from build123d import *

# Parameters (mm, degrees)
BOX035_W          = 6
BOX035_H          = 15
BOX035_DEPTH      = 3
CYLINDER018_R     = 2
CYLINDER018_DEPTH = 50
BOX_W             = 15
BOX_H             = 15
BOX_DEPTH         = 58
BOX038_W          = 80
BOX038_H          = 5
BOX038_DEPTH      = 58
BOX039_W          = 80
BOX039_H          = 90
BOX039_DEPTH      = 4


with BuildPart() as nut_hole:
    # Box035 → Box035 (new body)
    with BuildSketch(Plane(origin=(-8.5, 5, 15), x_dir=(1, 0, 0), z_dir=(0, 0, 1))):
        with Locations((3, 7.5)):
            Rectangle(BOX035_W, BOX035_H)
    extrude(amount=BOX035_DEPTH)


with BuildPart() as cylinder:
    # Cylinder018 → Cylinder018 (new body)
    with BuildSketch(Plane(origin=(-5.5, 12, 0), x_dir=(1, 0, 0), z_dir=(0, 0, 1))):
        Circle(CYLINDER018_R)
    extrude(amount=CYLINDER018_DEPTH)


with BuildPart() as cut:
    # Box → Box (new body)
    with BuildSketch(Plane(origin=(-13, 5, 0), x_dir=(1, 0, 0), z_dir=(0, 0, 1))):
        with Locations((7.5, 7.5)):
            Rectangle(BOX_W, BOX_H)
    extrude(amount=BOX_DEPTH)

    # Cut: cut Cylinder
    add(cylinder.part, mode=Mode.SUBTRACT)


with BuildPart() as cut037:
    # Cut037 base: copy of Cut
    add(cut.part)

    # Cut037: cut Nut hole
    add(nut_hole.part, mode=Mode.SUBTRACT)


with BuildPart() as cut037_1:
    # Cut037 placement: moved
    add(cut037.part.moved(Location((-22, 0, 0))))


with BuildPart() as cut038:
    # Cut038 base: copy of Cut
    add(cut.part)

    # Cut038: cut Nut hole
    add(nut_hole.part, mode=Mode.SUBTRACT)


with BuildPart() as cut038_1:
    # Cut038 placement: moved
    add(cut038.part.moved(Location((43, 0, 0))))


with BuildPart() as extension_supports:
    # Cut039 base: copy of Cut
    add(cut.part)

    # Cut039: cut Nut hole
    add(nut_hole.part, mode=Mode.SUBTRACT)


with BuildPart() as extension_supports_1:
    # Cut039 placement: moved
    add(extension_supports.part.moved(Location((10, 70, 0))))

    # Fusion082: union Cut037, Cut038
    add(cut037_1.part)
    add(cut038_1.part)


with BuildPart() as cube002:
    # Box038 → Box038 (new body)
    with BuildSketch(Plane(origin=(-35, 0, 0), x_dir=(1, 0, 0), z_dir=(0, 0, 1))):
        with Locations((40, 2.5)):
            Rectangle(BOX038_W, BOX038_H)
    extrude(amount=BOX038_DEPTH)


with BuildPart() as fusion084:
    # Box039 → Box039 (new body)
    with BuildSketch(Plane(origin=(-35, 0, 58), x_dir=(1, 0, 0), z_dir=(0, 0, 1))):
        with Locations((40, 45)):
            Rectangle(BOX039_W, BOX039_H)
    extrude(amount=BOX039_DEPTH)

    # Fusion081: union Cube002
    add(cube002.part)

    # Fusion084: union Extension supports
    add(extension_supports_1.part)


solid = fusion084.part
Design review of the part built by this model. Coordinates are the model's own, in mm. A direction names the side the tool comes from. Round coordinates to 2 decimals unless told otherwise and drop trailing zeros. Loops run counter-clockwise (first coordinate to the right, second up) from the corner with the lowest first, then second, coordinate; pieces in that order, holes last. Notation, with made-up numbers: (14, 14) - (54, 14) arc R28 ccw to (54, 38) - close; hole circle Ø10 at (35, 0). An arc over 180 degrees is marked (long way). One line per item, written item: value. Start each with the question number.
1) For faces 4 (the flat face through (4, 75, 29)), 5 (the cylindrical face through (37.24, 13.983, 7.395)), 6 (the flat face through (30, 12, 29)), list the 3-axis set-ups (+Z, -Z, +X, -X, +Y, -Y) from which the entire face can be reached by the end or side of a thin tool; tool diameter is ignored.
2) Consider section D-D on y = 8. Give the boundary of the cut face in (x, z).
3) Draft analysis for pull direction Z (two halves, no side actions). For faces 1 (the cylindrical face through (-25.592, 12.601, 7.395)), 2 (the flat face through (4.4, 84.3, 0)), 3 (the flat face through (4.5, 84.3, 15)), state which applies: +Z half, -Z half, draft (parallel to the pull), parting line (faces both ways), or undercut.
4) To check wall thickness, follow L1, parallel to X at y = 12, z = 29; L2, parallel to Y at x = -27.5, z = 28.5; L3, parallel to X at y = 15, z = 50.5. State the ranges of each line that lie inside material, in increasing order. Write a range as from..to.
5) Consider section A-A on z = 9.5. Give the boundary of the cut face in (x, y), then the cut area to 3 significant figures.
6) Insertion check: pin 1 Ø8 at (x, y) = (3.5, 37.5) entering from -Z; pin 2 Ø4.5 at (y, z) = (80, 20.5) entering from -X; pin 3 Ø2.5 at (x, y) = (-27.5, 12) entering from -Z. Each pin has a flat end and moves straight along its axis. Give the tip position at first contact, or say it passes through.
7) Consider section C-C on x = 37.5. Give the boundary of the cut face in (y, z), then the cut area to 3 significant figures.
8) Consider section B-B on z = 53. Give the boundary of the cut face in (x, y).
Reported:
1. face 4: -Z, +X, -X
1. face 5: -Z
1. face 6: -Z, +Y
2. outline: (-35, 0) - (-20, 0) - (-20, 58) - (30, 58) - (30, 0) - (45, 0) - (45, 62) - (-35, 62) - close; hole (-30.5, 15) - (-24.5, 15) - (-24.5, 18) - (-30.5, 18) - close; hole (34.5, 15) - (40.5, 15) - (40.5, 18) - (34.5, 18) - close
3. face 1: draft
3. face 2: -Z half
3. face 3: undercut
4. L1: x = -35..-29.5, -25.5..-20, 30..35.5, 39.5..45
4. L2: y = 0..10, 14..20
4. L3: x = -35..-20, 30..45
5. outline: (-35, 0) - (45, 0) - (45, 20) - (30, 20) - (30, 5) - (-20, 5) - (-20, 20) - (-35, 20) - close; (-3, 75) - (12, 75) - (12, 90) - (-3, 90) - close; hole circle Ø4 at (-27.5, 12); hole circle Ø4 at (4.5, 82); hole circle Ø4 at (37.5, 12)
5. area: 1,040 mm^2
6. pin 1: stops at z = 58
6. pin 2: stops at x = -3
6. pin 3: stops at z = 50
7. outline: (0, 0) - (10, 0) - (10, 15) - (5, 15) - (5, 18) - (10, 18) - (10, 50) - (14, 50) - (14, 18) - (20, 18) - (20, 58) - (90, 58) - (90, 62) - (0, 62) - close; (14, 0) - (20, 0) - (20, 15) - (14, 15) - close
7. area: 1,290 mm^2
8. outline: (-35, 0) - (45, 0) - (45, 20) - (30, 20) - (30, 5) - (-20, 5) - (-20, 20) - (-35, 20) - close; (-3, 75) - (12, 75) - (12, 90) - (-3, 90) - close
